```python
from build123d import *

# Parameters (mm, degrees)
F0_W      = 69.85
F0_H      = 44.45
F1_DEPTH  = 12.7
F2_T      = -6.35
F3_R      = 3.81
F4_R      = 2.54
F5_R      = 1.524
F5_R_2    = 1.8415
F6_DEPTH  = 4.572
F7_R      = 1.905
F8_DEPTH  = 6.35
F9_R      = 2.54
F10_DEPTH = 6.35
F12_DEPTH = 3.175


# Not quite as in the source:
# - a feature names something its author has since deleted; it is built from what else it names


with BuildPart() as f1:
    # F0 (on Front) → F1 (new body)
    with BuildSketch(Plane.XZ):
        Rectangle(F0_W, F0_H)
    extrude(amount=F1_DEPTH)

    # F2
    f2_openings = [f1.faces().sort_by_distance(p)[0] for p in [
        (0, 0, 0),
    ]]
    offset(amount=F2_T, openings=f2_openings)

    # F3
    f3_edges = [f1.edges().sort_by_distance(p)[0] for p in [
        (34.925, -6.35, -22.225),
        (34.925, -12.7, 0),
        (0, -12.7, -22.225),
        (-34.925, -12.7, 0),
        (0, -12.7, 22.225),
        (-34.925, -6.35, 22.225),
        (34.925, -6.35, 22.225),
        (-34.925, -6.35, -22.225),
    ]]
    fillet(f3_edges, radius=F3_R)

    # F4
    f4_edges = [f1.edges().sort_by_distance(p)[0] for p in [
        (-28.575, -6.35, 0),
        (0, -6.35, -15.875),
        (28.575, -6.35, 0),
        (0, -6.35, 15.875),
        (-28.575, -3.175, -15.875),
        (28.575, -3.175, -15.875),
        (28.575, -3.175, 15.875),
        (-28.575, -3.175, 15.875),
    ]]
    fillet(f4_edges, radius=F4_R)

    # F5 (on face) → F6 (join)
    with BuildSketch(Plane(origin=(0, 0, 0), x_dir=(-1, 0, 0), z_dir=(0, 1, 0))):
        with Locations((31.115, 18.415)):
            Circle(F5_R)
        with Locations((-31.115, -18.415)):
            Circle(F5_R_2)
    extrude(amount=F6_DEPTH)

    # F7 (on face) → F8 (cut, through all)
    with BuildSketch(Plane(origin=(0, -6.35, 0), x_dir=(-1, 0, 0), z_dir=(0, 1, 0))):
        with Locations((20.32, 0)):
            Circle(F7_R)
        with Locations((-17.78, 0)):
            Circle(F7_R)
    extrude(amount=-F8_DEPTH, mode=Mode.SUBTRACT)

    # F9 (on face) → F10 (cut, through all)
    with BuildSketch(Plane.XY.offset(22.225)):
        with Locations((-5.08, 0)):
            Circle(F9_R)
        with Locations((21.59, 0)):
            Circle(F9_R)
    extrude(amount=-F10_DEPTH, mode=Mode.SUBTRACT)

    # F11 (on face) → F12 (cut)
    with BuildSketch(Plane(origin=(0, 0, 15.875), x_dir=(1, 0, 0), z_dir=(0, 0, -1))):
        with BuildLine():
            add(Edge.make_bspline(
                [(-8.89, 0), (-8.89, -1.6497783942), (-3.175, -0.8248891971), (2.54, 0), (-3.175, 0.8248891971), (-8.89, 1.6497783942), (-8.89, 0)],
                knots=[0, 0, 0, 2.0943951024, 2.0943951024, 4.1887902048, 4.1887902048, 6.2831853072, 6.2831853072, 6.2831853072], degree=2, weights=[1, 0.5, 1, 0.5, 1, 0.5, 1]))
        make_face()
        with BuildLine():
            add(Edge.make_bspline(
                [(17.78, 0), (17.78, -1.6497783942), (23.495, -0.8248891971), (29.21, 0), (23.495, 0.8248891971), (17.78, 1.6497783942), (17.78, 0)],
                knots=[0, 0, 0, 2.0943951024, 2.0943951024, 4.1887902048, 4.1887902048, 6.2831853072, 6.2831853072, 6.2831853072], degree=2, weights=[1, 0.5, 1, 0.5, 1, 0.5, 1]))
        make_face()
    extrude(amount=-F12_DEPTH, mode=Mode.SUBTRACT)


solid = f1.part
```
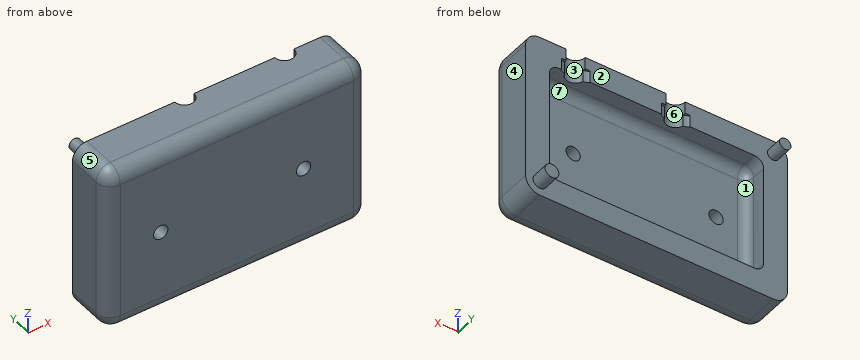
Part model, mm, in its own coordinate system. Face numbers are marked on the shaded views. A direction names the side the tool comes from. Round coordinates to 2 decimals unless told otherwise and drop trailing zeros. Loops run counter-clockwise (first coordinate to the right, second up) from the corner with the lowest first, then second, coordinate; pieces in that order, holes last.
Item 1: Cut at C-C, the plane z = 8. Give the cut face in (x, y) (3 decimals).
Item 2: Drop flat-ended pins along their axis: P1, Ø13.5, axis at x = 14.5, z = -7.5, coming from the +Y side; P2, Ø5, axis at x = 13, z = 18.5, coming from the +Y side; P3, Ø3, axis at x = 21, z = -8, coming from the +Y side; P4, Ø2.5, axis at x = -20.32, z = 0, coming from the -Y side. Give the stop position or say it passes through.
Item 3: Mould opens along Z. For the marked faces 5, 6 and 7 say: +Z half, -Z half, draft (parallel to the pull), parting line (faces both ways), or undercut.
Item 4: Cut at B-B, the plane x = 3. Give the cut face in (y, z) (3 decimals), then the cut area to 3 significant figures.
Item 5: Cut at A-A, the plane x = -20.32. Give the cut face in (y, z) (3 decimals), then the cut area to 3 significant figures.
Item 6: Drill centre lines: line 1 (Z direction, x = -20.32, y = -8) (3 decimals); line 2 (X direction, y = -1, z = 12) (3 decimals); line 3 (Y direction, x = 25, z = -7.5). Where is each one in solid material? Low to high.
Item 7: 3-axis set-ups, long thin cutter, end or side, ignore diameter. For the marked faces 1, 2, 3 and 4: which of +Z, -Z, +X, -X, +Y, -Y reach the whole face in a straight line?
A:
1. outline: (-34.925, -8.89) arc R3.81 ccw to (-31.115, -12.7) - (31.115, -12.7) arc R3.81 ccw to (34.925, -8.89) - (34.925, 0) - (28.575, 0) - (28.575, -3.81) arc R2.54 cw to (26.035, -6.35) - (-26.035, -6.35) arc R2.54 cw to (-28.575, -3.81) - (-28.575, 0) - (-34.925, 0) - close
2. P1: stops at y = -6.18
2. P2: stops at y = 0
2. P3: stops at y = -6.35
2. P4: passes through
3. face 5: +Z half
3. face 6: draft
3. face 7: undercut
4. outline: (-12.7, -18.415) arc R3.81 ccw to (-8.89, -22.225) - (0, -22.225) - (0, -15.875) - (-3.81, -15.875) arc R2.54 cw to (-6.35, -13.335) - (-6.35, 13.335) arc R2.54 cw to (-3.81, 15.875) - (0, 15.875) - (0, 22.225) - (-8.89, 22.225) arc R3.81 ccw to (-12.7, 18.415) - close
4. area: 359 mm2
5. outline: (-12.7, -18.415) arc R3.81 ccw to (-8.89, -22.225) - (0, -22.225) - (0, -15.875) - (-3.81, -15.875) arc R2.54 cw to (-6.35, -13.335) - (-6.35, -1.905) - (-12.7, -1.905) - close; (-12.7, 1.905) - (-6.35, 1.905) - (-6.35, 13.335) arc R2.54 cw to (-3.81, 15.875) - (0, 15.875) - (0, 22.225) - (-8.89, 22.225) arc R3.81 ccw to (-12.7, 18.415) - close
5. area: 335 mm2
6. line 1: z = -22.225 to -1.905, 1.905 to 22.225
6. line 2: x = -34.925 to -28.575, 28.575 to 34.925
6. line 3: y = -12.7 to -6.35
7. face 1: +Y
7. face 2: +Z, -Z, +X, +Y
7. face 3: +Z, +Y
7. face 4: +Z, -Z, +X, +Y, -Y
